```python
from build123d import *

# Parameters (mm, degrees)
SKETCH_1_R               = 15
SKETCH_1_R_2             = 6
SKETCH_1_R_3             = 1.65
EXTRUDE_1_DEPTH          = 10
SKETCH_2_R               = 1.65
CUT_EXTRUDE_1_DEPTH      = 24.452078799
PATTERN_CIRCULAR_1_COUNT = 3


with BuildPart() as part:
    # ｽｹｯﾁ1 → ﾎﾞｽ - 押し出し1 (new body)
    with BuildSketch(Plane(origin=(0, 0, 0), x_dir=(0, 0, -1), z_dir=(1, 0, 0))):
        Circle(SKETCH_1_R)
        Circle(SKETCH_1_R_2, mode=Mode.SUBTRACT)
        with Locations((-10, 0)):
            Circle(SKETCH_1_R_3, mode=Mode.SUBTRACT)
        with Locations(Location((10, 0, 0), (0, 0, 180))):
            Circle(SKETCH_1_R_3, mode=Mode.SUBTRACT)
    extrude(amount=EXTRUDE_1_DEPTH)

    # ｽｹｯﾁ2 → ｶｯﾄ - 押し出し1 (cut, through all)
    with BuildSketch(Plane(origin=(0, 0, 0), x_dir=(1, 0, 0), z_dir=(0, 1, 0))):
        with Locations(Location((5, 0, 0), (0, 0, 90))):
            Circle(SKETCH_2_R)
    cut_extrude_1 = extrude(amount=CUT_EXTRUDE_1_DEPTH, mode=Mode.SUBTRACT)

    # 円形ﾊﾟﾀｰﾝ1: ｶｯﾄ - 押し出し1 ×3 about axis
    pattern_circular_1_axis = Axis((10, 0, 0), (1, 0, 0))
    for i in range(1, PATTERN_CIRCULAR_1_COUNT):
        add(cut_extrude_1.rotate(pattern_circular_1_axis, i * 360 / PATTERN_CIRCULAR_1_COUNT), mode=Mode.SUBTRACT)


solid = part.part
```
Design review of the part built by this model. Coordinates are the model's own, in mm. Coordinates: 2 decimals unless noted, no trailing zeros. Loops run counter-clockwise (first coordinate to the right, second up) from the corner with the lowest first, then second, coordinate; pieces in that order, holes last. Notation, with made-up numbers: (23.5, 65.5) - (33.5, 65.5) arc R14 ccw to (33.5, 83.5) - close; hole circle Ø9 at (-5, 17). An arc over 180 degrees is marked (long way). Use CSV: the item, a comma, the result in double quotes. Start each with the question number.
1) Consider section D-D on y = 5. Write out the cut boundary in (x, z).
2) For pin 1 Ø4 at (x, z) = (3, 1) entering from +Y; pin 2 Ø1 at (x, y) = (6, 10) entering from -Z; pin 3 Ø6 at (x, y) = (7.5, -6.5) entering from -Z; pin 4 Ø1.5 at (x, y) = (6, 9) entering from +Z, all flat-tipped, find the tip position at first contact; note any pin that passes through.
3) Consider section A-A on y = 0. Write out the cut boundary in (x, z), then the cut area to 3 significant figures.
4) Consider section C-C on x = 5.75. Write out the cut boundary in (y, z).
5) Wall thickness on L1, parallel to Y at x = 4, z = 10; L2, parallel to Y at x = 7, z = 0; L3, parallel to Y at x = 3, z = 2.5: over which ranges is each line inside the solid? List them lowest first. Write a range as from..to.
6) Consider section B-B on z = 0. Write out the cut boundary in (x, y), then the cut area to 3 significant figures.
7) The part is to be moulded in two halves that separate along Y. For faces 1 (the cylindrical face through (6.6, 10.3, 0.4)), 2 (the cylindrical face through (4.93, 0.632, -8.476)), 3 (the cylindrical face through (4.93, 0.66, 14.985)), 4 (the cylindrical face through (4.93, -0.632, 8.476)), say which applies: +Y half, -Y half, draft (parallel to the pull), parting line (faces both ways), or undercut.
Geometry says:
1,outline,"(0, -14.14) - (10, -14.14) - (10, -3.32) - (0, -3.32) - close; (0, 3.32) - (10, 3.32) - (10, 14.14) - (0, 14.14) - close"
2,pin 1,"y = 15"
2,pin 2,"z = -11.61"
2,pin 3,"z = -14.59"
2,pin 4,"z = 12.53"
3,outline,"(0, -15) - (10, -15) - (10, -11.65) - (0, -11.65) - close; (0, -8.35) - (10, -8.35) - (10, -6) - (0, -6) - close; (0, 6) - (10, 6) - (10, 8.35) - (0, 8.35) - close; (0, 11.65) - (10, 11.65) - (10, 15) - (0, 15) - close"
3,area,"114 mm^2"
4,outline,"(-8.74, -12.19) - (-4.18, -4.3) arc R6 cw to (-4.18, 4.3) - (-8.74, 12.19) arc R15 ccw to start; (-6.19, -13.66) arc R15 ccw to (14.93, -1.47) - (5.82, -1.47) arc R6 cw to (-1.64, -5.77) - close; (-6.19, 13.66) - (-1.64, 5.77) arc R6 cw to (5.82, 1.47) - (14.93, 1.47) arc R15 ccw to start; hole circle Ø3.3 at (0, -10); hole circle Ø3.3 at (0, 10)"
5,L1,"-11.18..-7.29, -4.26..-1.65, 1.65..11.18"
5,L2,"-15..-6, 6..15"
5,L3,"-14.79..-5.45, 5.45..14.79"
6,outline,"(0, -15) - (10, -15) - (10, -6) - (0, -6) - close; (0, 6) - (3.35, 6) - (3.35, 15) - (0, 15) - close; (6.65, 6) - (10, 6) - (10, 15) - (6.65, 15) - close"
6,area,"150 mm^2"
7,face 1,"draft"
7,face 2,"undercut"
7,face 3,"parting line"
7,face 4,"undercut"
